Geometry check sheet. Reference: the model listing, model coordinates, mm. A direction names the side the tool comes from. Round coordinates to 2 decimals unless told otherwise and drop trailing zeros. Order: outer loops, then holes, each group sorted by start corner. A loop starts at its lowest first (then second) coordinate and runs counter-clockwise, first axis right, second up. Notation, with made-up numbers: (79, 48.5) -> (94, 48.5) arc R20 cw to (94, 55.5) -> close; hole circle Ø4 at (67.5, 38.25). An arc over 180 degrees is marked (long way). Use a Markdown table: item, result. Add a question column.
Item 1: Mould release check, pull along Z, two halves, no side actions. Record for faces 1 (the cylindrical face through (30, -1, 27)), 2 (the cylindrical face through (30, -95, 29)), 3 (the flat face through (60, -48, 25)), 4 (the cylindrical face through (30.42, -56.55, 33.04)): pulls with the +Z half, pulls with the -Z half, needs draft (parallel to the pull), parting line crosses it, or undercut.
Item 2: Sectioned sample at D-D, the plane y = -81.5. Record the cut outline in (x, z).
Item 3: Sectioned sample at B-B, the plane y = -34.5. Record the cut outline in (x, z).
Item 4: Gauge pin test, flat ends, axial feed: pin 1 Ø23.5 at (x, y) = (19.5, -35.5) entering from +Z; pin 2 Ø2.5 at (x, z) = (17, 6.5) entering from -Y; pin 3 Ø1.5 at (y, z) = (-30, 47) entering from -X; pin 4 Ø10 at (y, z) = (-27, 14) entering from -X. Record the tip position at first contact, or that the pin passes through.
Item 5: Material ranges on probe 1 along Z at (x, y) = (53, -4.5); probe 2 along Z at (x, y) = (30.5, -11.5); probe 3 along Z at (x, y) = (43.5, -26), recorded low to high. Write a range as [from, to].
Item 6: Set-up check for faces 5 (the flat face through (30, -80, 7)), 6 (the flat face through (29.58, -6.956, 62.218)), 7 (the flat face through (30, -35, 24)), 8 (the flat face through (29.58, -83.83, 39.52)): record each of +Z, -Z, +X, -X, +Y, -Y from which the full face is reachable in a straight line by a thin tool's end or side.
Item 7: Sectioned sample at C-C, the plane z = 19. Record the cut outline in (x, y), and give its area (3 significant figures).
from build123d import *

# Parameters (mm, degrees)
F1_DEPTH = 60
F2_R     = 4.99999


# Not quite as in the source:
# - a fillet or chamfer is up to 0.001 mm smaller than in the source, because OpenCascade refuses the exact size


with BuildPart() as f1:
    # F0 (on Right) → F1 (new body)
    with BuildSketch(Plane.YZ):
        Polygon((-80, 0), (0, 0), (0, 5), (-70, 5), (-70, 24), (0, 24), (0, 29), (-80, 29), (-80, 14), align=None)
        with BuildLine():
            ThreePointArc((-85.1303021499, 43.0953893118), (-94.7721162952, 26.395277335), (-80, 14))
            Line((-80, 14), (-80, 29))
            Line((-80, 29), (-82.5651510749, 36.0476946559))
            Line((-82.5651510749, 36.0476946559), (-85.1303021499, 43.0953893118))
        make_face()
        Polygon((-82.5651510749, 36.0476946559), (-80, 29), (-4.8245903371, 56.3616114661), (-7.3897414121, 63.4093061219), align=None)
    extrude(amount=F1_DEPTH)

    # F2 (radius 5 in the source; OpenCascade refuses exactly that, so slightly less here)
    f2_edges = [f1.edges().sort_by_distance(p)[0] for p in [
        (30, -80, 29),
        (30, -80, 14),
        (30, -80, 0),
        (30, 0, 0),
        (30, 0, 29),
        (30, -4.82459, 56.361611),
    ]]
    fillet(f2_edges, radius=F2_R)


solid = f1.part
Found:
| question | item | result |
|---|---|---|
| 1 | face 1 | pulls with the +Z half |
| 1 | face 2 | parting line crosses it |
| 1 | face 3 | needs draft |
| 1 | face 4 | undercut |
| 2 | outline | (0, 13.21) -> (60, 13.21) -> (60, 36.44) -> (0, 36.44) -> close |
| 3 | outline | (0, 0) -> (60, 0) -> (60, 5) -> (0, 5) -> close; (0, 24) -> (60, 24) -> (60, 29) -> (0, 29) -> close; (0, 45.56) -> (60, 45.56) -> (60, 53.54) -> (0, 53.54) -> close |
| 4 | pin 1 | stops at z = 57.45 |
| 4 | pin 2 | stops at y = -80 |
| 4 | pin 3 | stops at x = 0 |
| 4 | pin 4 | passes through |
| 5 | probe 1 | z = [0.03, 5], [24, 28.97] |
| 5 | probe 2 | z = [0, 5], [24, 29], [53.93, 61.91] |
| 5 | probe 3 | z = [0, 5], [24, 29], [48.65, 56.64] |
| 6 | face 5 | -Z, +X, -X, -Y |
| 6 | face 6 | +Z, +X, -X, +Y |
| 6 | face 7 | +X, -X, +Y |
| 6 | face 8 | +Z, +X, -X |
| 7 | outline | (0, -91.18) -> (60, -91.18) -> (60, -70) -> (0, -70) -> close |
| 7 | area | 1,270 mm2 |
